Check sheet for the drawn part. Datum: minimum x, y, z corner. Units: mm. Give positions to 0.01 mm unless a question says otherwise; leave off trailing zeros. Order: outer loops, then holes, each group sorted by start corner. A loop starts at its lowest first (then second) coordinate and runs counter-clockwise, first axis right, second up.
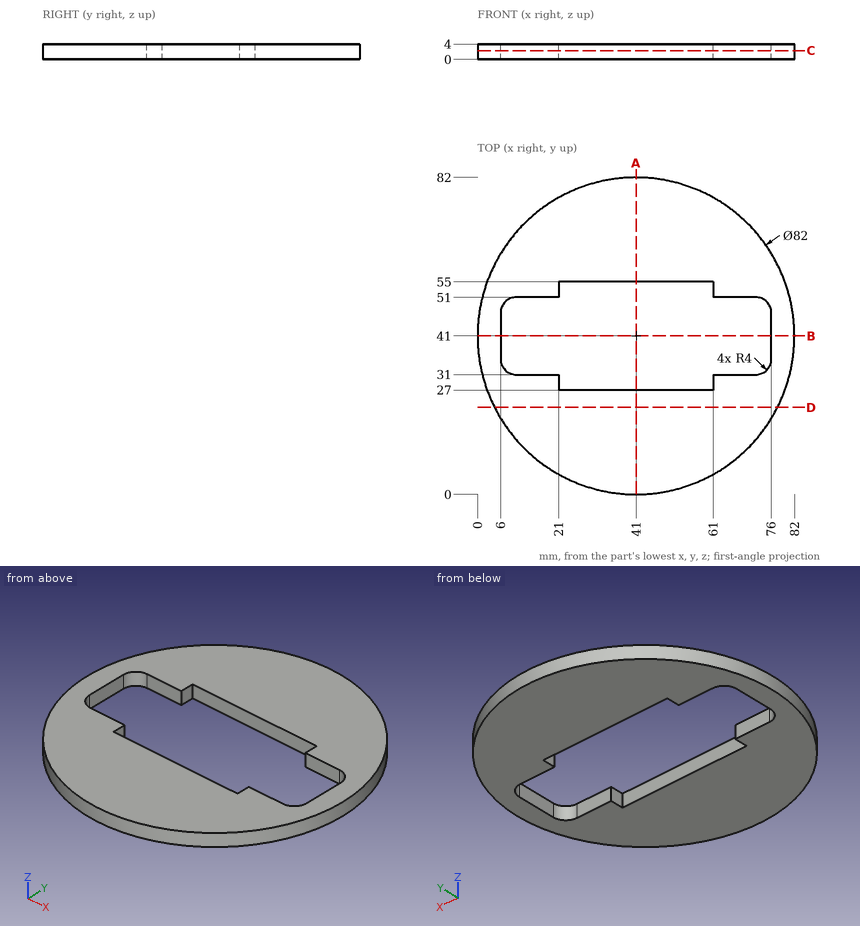
Item 1: Gauge pin test, flat ends, axial feed: pin 1 (1.2 mm diameter, centred on y = 42.5, z = 1.5, fed in from -X); pin 2 (1 mm diameter, centred on x = 59.5, z = 1, fed in from -Y); pin 3 (1.2 mm diameter, centred on x = 67, z = 1, fed in from -Y); pin 4 (8 mm diameter, centred on x = 73.5, y = 13, fed in from -Z). Record the tip position at first contact, or that the pin passes through.
Reported:
pin 1: stops at x = 0.01
pin 2: stops at y = 4.16
pin 3: stops at y = 8.82
pin 4: stops at z = 0
Item 2: Sectioned sample at D-D (y = 22.5). Enter the section's corners in (x, z).
Reported:
outline: (4.41, 0) - (77.59, 0) - (77.59, 4) - (4.41, 4) - close
Item 3: Sectioned sample at C-C (z = 2.3). Enter the section's corners in (x, y), and give its area (3 significant figures).
Reported:
outline: circle Ø82 at (41, 41); hole (6, 35) arc R4 ccw to (10, 31) - (21, 31) - (21, 27) - (61, 27) - (61, 31) - (72, 31) arc R4 ccw to (76, 35) - (76, 47) arc R4 ccw to (72, 51) - (61, 51) - (61, 55) - (21, 55) - (21, 51) - (10, 51) arc R4 ccw to (6, 47) - close
area: 3,570 mm2
Item 4: Sectioned sample at B-B (y = 41). Enter the section's corners in (x, z).
Reported:
outline: (0, 0) - (6, 0) - (6, 4) - (0, 4) - close; (76, 0) - (82, 0) - (82, 4) - (76, 4) - close
Item 5: Sectioned sample at A-A (x = 41). Enter the section's corners in (y, z), and give its area (3 significant figures).
Reported:
outline: (0, 0) - (27, 0) - (27, 4) - (0, 4) - close; (55, 0) - (82, 0) - (82, 4) - (55, 4) - close
area: 216 mm2
Item 6: Scan lines: L1, parallel to Y at x = 27, z = 1.7; L2, parallel to Y at x = 68, z = 0.4; L3, parallel to X at y = 66, z = 2.1. Record each from-to range of solid material in increasing order.
Reported:
L1: y = 2.46 to 27, 55 to 79.54
L2: y = 10.15 to 31, 51 to 71.85
L3: x = 8.5 to 73.5
